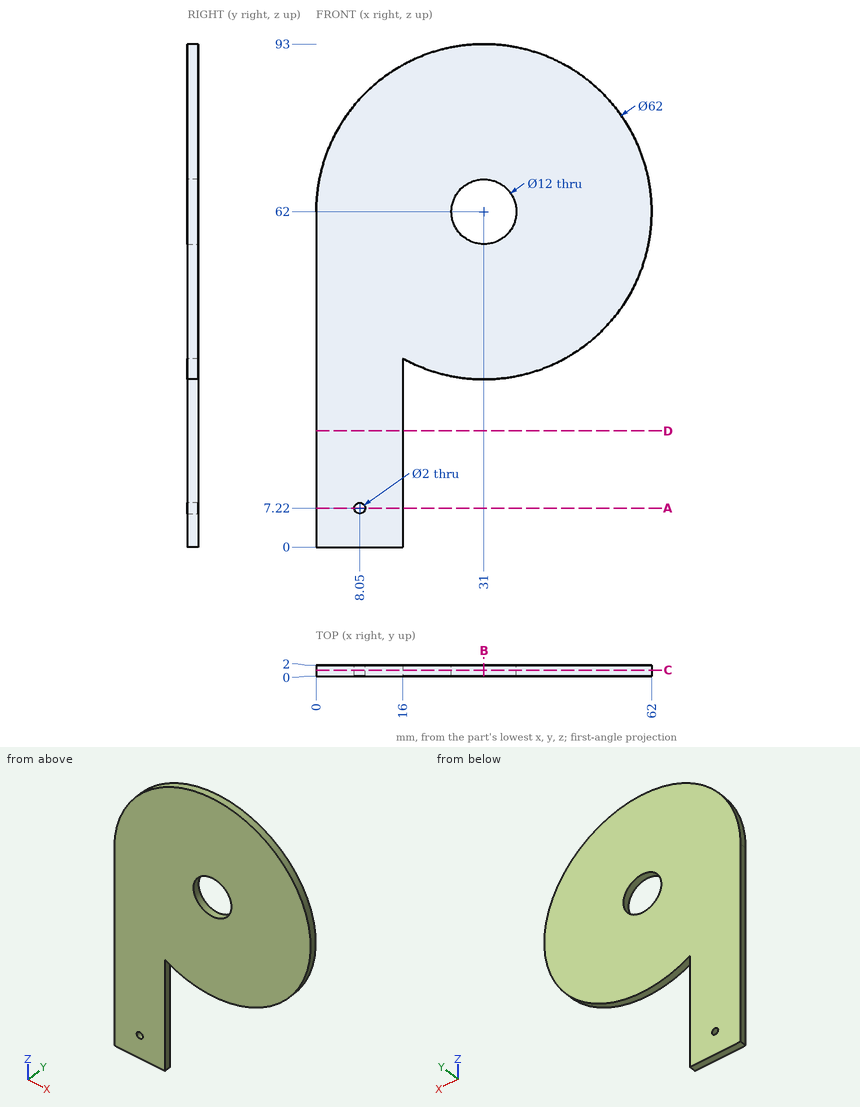
Design review of the part shown in the three views and the two pictorial views. Dimensions are in mm from the part's minimum x, y and z. Give positions to 0.01 mm unless a question says otherwise; leave off trailing zeros. Loops run counter-clockwise (first coordinate to the right, second up) from the corner with the lowest first, then second, coordinate; pieces in that order, holes last. Notation, with made-up numbers: (-10.75, 88) -> (17.25, 88) arc R5 cw to (17.25, 93) -> close; hole circle Ø8 at (86, -36). An arc over 180 degrees is marked (long way). One line per item, written item: value.
Q1. For pin 1 Ø8 at (x, z) = (54.5, 33) entering from -Y; pin 2 Ø1 at (x, z) = (14.5, 70) entering from -Y, all flat-tipped, find the tip position at first contact; note any pin that passes through.
Numbers:
pin 1: passes through
pin 2: stops at y = 0
Q2. For L1, parallel to X at y = 1.45, z = 62; L2, parallel to X at y = 0.95, z = 7.22; L3, parallel to X at y = 1.25, z = 28, list the stretches that pass through material, from the lowest coordinate up.
Numbers:
L1: x = 0 to 25, 37 to 62
L2: x = 0 to 7.05, 9.05 to 16
L3: x = 0 to 16
Q3. We need section D-D on z = 21.5. Give the boundary of the cut face in (x, y), and give its area (3 significant figures).
Numbers:
outline: (0, 0) -> (16, 0) -> (16, 2) -> (0, 2) -> close
area: 32.0 mm^2
Q4. We need section B-B on x = 31. Give the boundary of the cut face in (y, z), and give its area (3 significant figures).
Numbers:
outline: (0, 31) -> (2, 31) -> (2, 56) -> (0, 56) -> close; (0, 68) -> (2, 68) -> (2, 93) -> (0, 93) -> close
area: 100 mm^2
Q5. We need section A-A on z = 7.22. Give the boundary of the cut face in (x, y), and give its area (3 significant figures).
Numbers:
outline: (0, 0) -> (7.05, 0) -> (7.05, 2) -> (0, 2) -> close; (9.05, 0) -> (16, 0) -> (16, 2) -> (9.05, 2) -> close
area: 28.0 mm^2
Q6. We need section C-C on y = 1.1. Give the boundary of the cut face in (x, z), and give its area (3 significant figures).
Numbers:
outline: (0, 0) -> (16, 0) -> (16, 34.87) arc R31 ccw (long way) to (0, 62) -> close; hole circle Ø2 at (8.05, 7.22); hole circle Ø12 at (31, 62)
area: 3,590 mm^2
